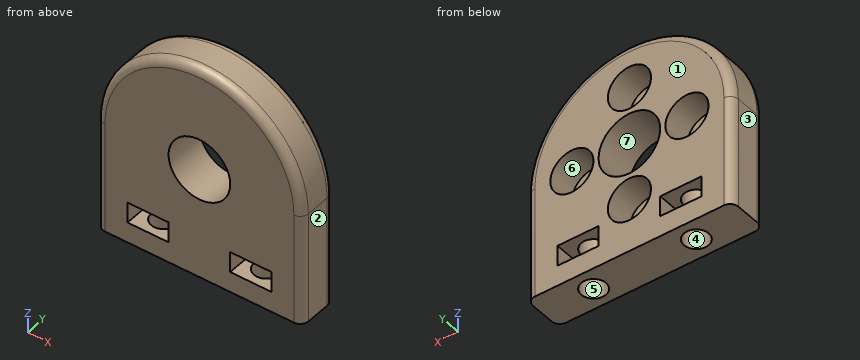
from build123d import *

# Parameters (mm, degrees)
SKETCH_R        = 7.5
PAD_DEPTH       = 10
SKETCH002_W     = 10
SKETCH002_H     = 5
POCKET001_DEPTH = 10.001
SKETCH003_R     = 3
POCKET002_DEPTH = 15
SKETCH001_R     = 5.25
POCKET_DEPTH    = 7
FILLET_R        = 2
FILLET001_R     = 2


with BuildPart() as part:
    # Sketch → Pad (new body)
    with BuildSketch(Plane.XZ):
        with BuildLine():
            Line((-25, 0), (-25, 27))
            ThreePointArc((25, 27), (0, 52), (-25, 27))
            Line((25, 27), (25, 0))
            Line((25, 0), (-25, 0))
        make_face()
        with Locations((0, 27)):
            Circle(SKETCH_R, mode=Mode.SUBTRACT)
    extrude(amount=PAD_DEPTH)

    # Sketch002 → Pocket001 (cut, through all)
    with BuildSketch(Plane.XZ.offset(10)):
        with Locations((-12.5, 7.5)):
            Rectangle(SKETCH002_W, SKETCH002_H)
        with Locations((12.5, 7.5)):
            Rectangle(SKETCH002_W, SKETCH002_H)
    extrude(amount=-POCKET001_DEPTH, mode=Mode.SUBTRACT)

    # Sketch003 (on Face2 of Pocket001) → Pocket002 (cut)
    with BuildSketch(Plane(origin=(0, 0, 0), x_dir=(1, 0, 0), z_dir=(0, 0, -1))):
        with Locations((-12.5, 5)):
            Circle(SKETCH003_R)
        with Locations((12.5, 5)):
            Circle(SKETCH003_R)
    extrude(amount=-POCKET002_DEPTH, mode=Mode.SUBTRACT)

    # Sketch001 (on Face6 of Pad) → Pocket (cut)
    with BuildSketch(Plane(origin=(0, 0, 0), x_dir=(1, 0, 0), z_dir=(0, 1, 0))):
        with Locations((14, -27)):
            Circle(SKETCH001_R)
        with Locations((0, -13)):
            Circle(SKETCH001_R)
        with Locations((0, -41)):
            Circle(SKETCH001_R)
        with Locations((-14, -27)):
            Circle(SKETCH001_R)
    extrude(amount=-POCKET_DEPTH, mode=Mode.SUBTRACT)

    # Fillet
    fillet_edges = [part.edges().sort_by_distance(p)[0] for p in [
        (-25, 0, 13.5),
    ]]
    fillet(fillet_edges, radius=FILLET_R)

    # Fillet001
    fillet001_edges = [part.edges().sort_by_distance(p)[0] for p in [
        (25, -10, 13.5),
    ]]
    fillet(fillet001_edges, radius=FILLET001_R)


solid = part.part
Build history of the part. All positions in model axes, mm. Face numbers are marked on the shaded views. A direction names the side the tool comes from. Round coordinates to 2 decimals unless told otherwise and drop trailing zeros. Use CSV: the item, a comma, the result in double quotes. Start each with the question number.
Q1. Saw through at A-A on y = -5. Count the separate pieces of the cut face and the enclosed holes in it, and give its area (3 significant figures).
Q2. Flat gauge pins, fed straight in: pin 1 Ø4 at (x, y) = (-9.5, -2) entering from +Z; pin 2 Ø5.5 at (x, y) = (12.5, -5) entering from -Z; pin 3 Ø3 at (x, y) = (-18, -7.5) entering from +Z. Where does each tip first touch, or does it go through?
Q3. Which spindle directions (+Z, -Z, +X, -X, +Y, -Y) get a long thin tool onto all of the face, cutting with end or side? Do the marked faces 5, 6 and 7. Say none if no direction does.
Q4. Drill centre lines: L1, parallel to X at y = -5, z = 2.8; L2, parallel to Z at x = 0, y = -3.75; L3, parallel to Y at x = -12.5, z = 13.55. Where is each one in solid material? Low to high.
Q5. Mould opens along X. For the marked faces 1, 2, 3 and 4 say: +X half, -X half, draft (parallel to the pull), parting line (faces both ways), or undercut.
Solutions:
1,separate pieces,"1"
1,enclosed holes,"5"
1,area,"1,590 mm^2"
2,pin 1,"stops at z = 50.85"
2,pin 2,"stops at z = 15"
2,pin 3,"stops at z = 45.78"
3,face 5,"-Z"
3,face 6,"+Y"
3,face 7,"+Y, -Y"
4,L1,"x = -25 to -15.5, -9.5 to 9.5, 15.5 to 25"
4,L2,"z = 0 to 7.75, 18.25 to 19.5, 34.5 to 35.75, 46.25 to 52"
4,L3,"y = -10 to -8, -2 to 0"
5,face 1,"draft"
5,face 2,"+X half"
5,face 3,"-X half"
5,face 4,"undercut"
